The model under review builds one solid part; all positions refer to its coordinate system, in mm. Coordinates: 2 decimals unless noted, no trailing zeros. Loops run counter-clockwise (first coordinate to the right, second up) from the corner with the lowest first, then second, coordinate; pieces in that order, holes last. Notation, with made-up numbers: (65.5, 79.5) - (89.5, 79.5) arc R18 ccw to (89.5, 83.5) - close; hole circle Ø10 at (2, 52). An arc over 180 degrees is marked (long way). Use a Markdown table: item, result. Add a question column.
1) To check wall thickness, follow L1, parallel to Y at x = 0, z = -0.15; L2, parallel to X at y = -4.75, z = -0.65; L3, parallel to X at y = -2.5, z = -1.75. State the ranges of each line that lie inside material, in increasing order. Write a range as [from, to].
2) Add section A-A, the plane x = 0. Give the boundary of the cut face in (y, z).
3) The part is to be moulded in two halves that separate along X. For faces 1 (the flat face through (6.5, -2.1, -1.95)), 2 (the cylindrical face through (-4.434, -3.4, -0.523)), 3 (the cylindrical face through (-1.29, 9.82, -0.96)), say which applies: pulls with the +X half, pulls with the -X half, needs draft (parallel to the pull), parting line crosses it, or undercut.
4) Add section D-D, the plane x = -8. Give the boundary of the cut face in (y, z).
5) Clearance check with flat-ended pins moving along their axes: pin 1 (1 mm diameter, centred on y = 7, z = -0.5, fed in from -X); pin 2 (1 mm diameter, centred on y = -7, z = -1, fed in from +X). State where each tip first meets the part, or that it passes through.
6) Add section C-C, the plane z = -0.7. Give the boundary of the cut face in (x, y), and give its area (3 significant figures).
```python
from build123d import *

# Parameters (mm, degrees)
SKETCH1_R                  = 9.906
BOSS_EXTRUDE1_DEPTH        = 1.95
F_97_0_44_DIAMETER_HOLE1_D = 11.176


# Read off the part's stored shape, not the designer's step: Cut-Sweep1
with BuildPart() as part:
    # Sketch1 → Boss-Extrude1 (new body)
    with BuildSketch(Plane.XY):
        Circle(SKETCH1_R)
    extrude(amount=-BOSS_EXTRUDE1_DEPTH)

    # #97 (0.44) Diameter Hole1 (through all)
    with Locations(Plane(origin=(0, 0, -1.95), x_dir=(-1, 0, 0), z_dir=(0, 0, -1))):
        with Locations((0, 0)):
            Hole(F_97_0_44_DIAMETER_HOLE1_D / 2)

    # Cut-Sweep1 outline → Cut-Sweep1 (revolve, cut)
    with BuildSketch(Plane.XZ):
        with BuildLine():
            ThreePointArc((6.477, -1.95), (6.216617928, -1.321382072), (5.588, -1.061))
            Line((5.588, -1.061), (5.588, -1.95))
            Line((5.588, -1.95), (6.477, -1.95))
        make_face()
    revolve(axis=Axis((0, 0, 0), (0, 0, 1)), mode=Mode.SUBTRACT)


solid = part.part
```
From the geometry:
| question | item | result |
|---|---|---|
| 1 | L1 | y = [-9.91, -5.59], [5.59, 9.91] |
| 1 | L2 | x = [-8.69, -2.94], [2.94, 8.69] |
| 1 | L3 | x = [-9.59, -5.95], [5.95, 9.59] |
| 2 | outline | (-9.91, -1.95) - (-6.48, -1.95) arc R0.89 cw to (-5.59, -1.06) - (-5.59, 0) - (-9.91, 0) - close; (5.59, -1.06) arc R0.89 cw to (6.48, -1.95) - (9.91, -1.95) - (9.91, 0) - (5.59, 0) - close |
| 3 | face 1 | needs draft |
| 3 | face 2 | undercut |
| 3 | face 3 | parting line crosses it |
| 4 | outline | (-5.84, -1.95) - (5.84, -1.95) - (5.84, 0) - (-5.84, 0) - close |
| 5 | pin 1 | stops at x = -7.48 |
| 5 | pin 2 | stops at x = 7.48 |
| 6 | outline | circle Ø19.81 at (0, 0); hole circle Ø11.18 at (0, 0) |
| 6 | area | 210 mm^2 |
